Model file for the job. Use its own axes, mm. Face numbers are marked on the shaded views. A direction names the side the tool comes from. Coordinates: 2 decimals unless noted, no trailing zeros. Order: outer loops, then holes, each group sorted by start corner. A loop starts at its lowest first (then second) coordinate and runs counter-clockwise, first axis right, second up. Notation, with made-up numbers: (88, 53.25) -> (106, 53.25) arc R29 ccw to (106, 83.25) -> close; hole circle Ø7 at (26.5, 25). An arc over 180 degrees is marked (long way). Write item = value, one per line. Start each with the question number.
Q1. Mould opens along X. For the marked faces 1, 2, 3 and 4 say: +X half, -X half, draft (parallel to the pull), parting line (faces both ways), or undercut.
Q2. Wall check: line 1 (Z direction, x = -7.7, y = -7.7); line 2 (X direction, y = -5.25, z = 3.5); line 3 (Y direction, x = 5, z = 2). Give the ranges that are in metal, low to high. Write a range as from..to.
Q3. 3-axis set-ups, long thin cutter, end or side, ignore diameter. For the marked faces 5, 6 and 7: which of +Z, -Z, +X, -X, +Y, -Y reach the whole face in a straight line?
Q4. Cut at B-B, the plane y = -7.7. List the corners of the cut face in (x, z).
Q5. Cut at A-A, the plane z = 3.35. Give the number of separate pieces and of enclosed holes in the cut face, plus the area to 3 significant figures.
Q6. Flat gauge pins, fed straight in: pin 1 (3 mm diameter, centred on x = -6.5, z = 5.5, fed in from +Y); pin 2 (8 mm diameter, centred on x = -1.5, y = 0.5, fed in from -Z); pin 3 (2 mm diameter, centred on x = -7.5, z = 1.5, fed in from +Y); pin 4 (2.5 mm diameter, centred on y = -7, z = 4, fed in from +X). Where does each tip first touch, or does it go through?
Q7. Cut at D-D, the plane y = -2.5. List the corners of the cut face in (x, z).
Q8. Cut at C-C, the plane z = 2. List the corners of the cut face in (x, y), plus the area to 3 significant figures.
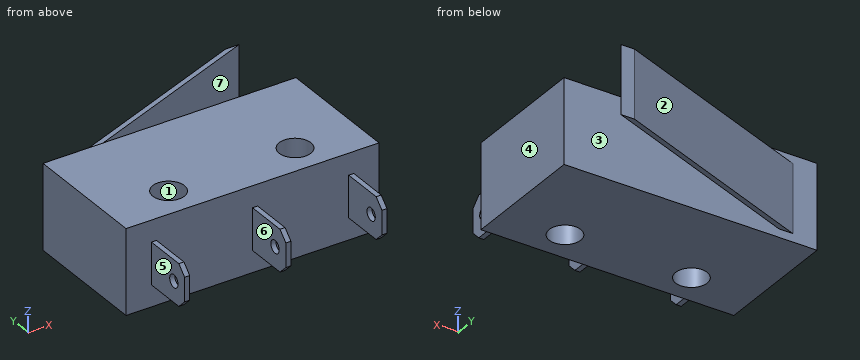
from build123d import *

# Parameters (mm, degrees)
F0_R     = 1.25
F1_DEPTH = 6.7
F2_W     = 0.4
F2_H     = 3.3
F3_W     = 1.1
F3_H     = 5.4
F6_R     = 0.5
F7_DEPTH = 25
F8_SIZE  = 0.7


with BuildPart() as f1:
    # F0 (on Top) → F1 (new body)
    with BuildSketch(Plane.XY):
        Polygon((-7, 5), (-10, 5), (-10, -5), (-8, -5), (0, -5), (8, -5), (10, -5), (10, 5), align=None)
        with Locations((-5, -2.5)):
            Circle(F0_R, mode=Mode.SUBTRACT)
        with Locations((5, -2.5)):
            Circle(F0_R, mode=Mode.SUBTRACT)
    extrude(amount=F1_DEPTH)

    # F4: sweep along a path in F0
    with BuildLine(Plane.XY) as f4_path:
        Line((-8, -5), (-8, -9))
    # F2 (on face) → F4 (sweep)
    with BuildSketch(Plane.XZ.offset(5)):
        with Locations((-7.8, 3.35)):
            Rectangle(F2_W, F2_H)
        with Locations((0.2, 3.35)):
            Rectangle(F2_W, F2_H)
        with Locations((7.8, 3.35)):
            Rectangle(F2_W, F2_H)
    sweep(path=f4_path.line)

    # F5: sweep along a path in F0
    with BuildLine(Plane.XY) as f5_path:
        Line((-7, 5), (9.7854103316, 11.5))
    # F3 (on face) → F5 (sweep)
    with BuildSketch(Plane(origin=(0, 5, 0), x_dir=(-1, 0, 0), z_dir=(0, 1, 0))):
        with Locations((7.55, 3.35)):
            Rectangle(F3_W, F3_H)
    sweep(path=f5_path.line)

    # F6 (on face) → F7 (cut)
    with BuildSketch(Plane.YZ.offset(8)):
        with Locations((-7.7, 3.35)):
            Circle(F6_R)
    extrude(amount=-F7_DEPTH, mode=Mode.SUBTRACT)

    # F8
    f8_edges = [f1.edges().sort_by_distance(p)[0] for p in [
        (-7.8, -9, 5),
        (0.2, -9, 5),
        (7.8, -9, 5),
        (-7.8, -9, 1.7),
        (0.2, -9, 1.7),
        (7.8, -9, 1.7),
    ]]
    chamfer(f8_edges, length=F8_SIZE)


solid = f1.part
Here are the results:
q1.face_1 = undercut
q1.face_2 = -X half
q1.face_3 = draft
q1.face_4 = +X half
q2.line_1 = 1.7..2.85, 3.85..5
q2.line_2 = -8..-7.6, 0..0.4, 7.6..8
q2.line_3 = -5..-3.75, -1.25..5, 9.65..10.07
q3.face_5 = +Z, -Z, -X, -Y
q3.face_6 = +Z, -Z, -Y
q3.face_7 = +Z, -Z, +X
q4.outline = (-8, 1.7) -> (-7.6, 1.7) -> (-7.6, 2.85) -> (-8, 2.85) -> close; (-8, 3.85) -> (-7.6, 3.85) -> (-7.6, 5) -> (-8, 5) -> close; (0, 1.7) -> (0.4, 1.7) -> (0.4, 2.85) -> (0, 2.85) -> close; (0, 3.85) -> (0.4, 3.85) -> (0.4, 5) -> (0, 5) -> close; (7.6, 1.7) -> (8, 1.7) -> (8, 2.85) -> (7.6, 2.85) -> close; (7.6, 3.85) -> (8, 3.85) -> (8, 5) -> (7.6, 5) -> close
q5.separate_pieces = 4
q5.enclosed_holes = 2
q5.area = 201 mm²
q6.pin_1 = 6.2
q6.pin_2 = 0
q6.pin_3 = 5.62
q6.pin_4 = 8
q7.outline = (-10, 0) -> (-6.25, 0) -> (-6.25, 6.7) -> (-10, 6.7) -> close; (-3.75, 0) -> (3.75, 0) -> (3.75, 6.7) -> (-3.75, 6.7) -> close; (6.25, 0) -> (10, 0) -> (10, 6.7) -> (6.25, 6.7) -> close
q8.outline = (-10, -5) -> (-8, -5) -> (-8, -8.6) -> (-7.6, -8.6) -> (-7.6, -5) -> (0, -5) -> (0, -8.6) -> (0.4, -8.6) -> (0.4, -5) -> (7.6, -5) -> (7.6, -8.6) -> (8, -8.6) -> (8, -5) -> (10, -5) -> (10, 5) -> (-7, 5) -> (9.79, 11.5) -> (8.69, 11.5) -> (-8.1, 5) -> (-10, 5) -> close; hole circle Ø2.5 at (-5, -2.5); hole circle Ø2.5 at (5, -2.5)
q8.area = 202 mm²
